Input: part model. Units: mm. Frame: model coordinates. A direction names the side the tool comes from. Coordinates: 2 decimals unless noted, no trailing zeros. Loops run counter-clockwise (first coordinate to the right, second up) from the corner with the lowest first, then second, coordinate; pieces in that order, holes last.
(1) Set-up query: faces 1 (the face through (-69.1, 19.27, -19.52)), 2 (the face through (62.2, 10, -26.2)). Return all of +Z, -Z, +X, -X, +Y, -Y with unobstructed straight access to the full face (end or side cutting, diameter ignored); none if empty.
(2) Line query: L1, parallel to X at y = 2.75, z = 24; L2, parallel to X at y = 2.5, z = 26; L3, parallel to Z at x = -60, y = 17.5. Output: solid intervals per line, ascending.
(3) Section B-B, the plane x = 43. Return loops of the section in (y, z).
(4) Mould query, pull axis Z, two halves, no side actions, for faces 3 (the face through (69.1, 29.14, 0.12)), 4 (the face through (60, 14, 19)), 5 (the face through (-57.8, 10, -26.2)), 6 (the face through (-1, 20, -20)). Classes: released by +Z, released by -Z, zero draft, split by the parting line, or undercut.
(5) Contact query for flat-ended pins moving along their axis: P1, Ø6, axis at x = 60, z = -24, coming from the +Y side; P2, Ø3, axis at x = -25, z = 17, coming from the +Y side; P3, Ø5, axis at x = 41.5, y = 14, coming from the -Z side; P4, Ø6, axis at x = -38, z = -5, coming from the -Y side. Output: stop coordinate, or through.
(6) Section A-A, the plane x = 60. Return loops of the section in (y, z).
(7) Section C-C, the plane z = 24. Give the number of separate pieces and of enclosed holes in the cut face, then the cut area to 3 significant figures.
```python
from build123d import *

# Parameters (mm, degrees)
SKETCH1_R           = 2.75
SKETCH1_W           = 130
SKETCH1_H           = 38
BOSS_EXTRUDE1_DEPTH = 10
SKETCH2_W           = 20
SKETCH2_H           = 20
BOSS_EXTRUDE3_DEPTH = 140
SKETCH3_R           = 5
CUT_EXTRUDE1_DEPTH  = 79.74007874
FILLET1_R           = 3


with BuildPart() as part:
    # Sketch1 → Boss-Extrude1 (new body)
    # profile 1 of 6: a face of its own
    with BuildSketch(Plane(origin=(0, 0, 0), x_dir=(1, 0, 0), z_dir=(0, 1, 0))):
        with BuildLine():
            Line((70, 30), (67, 30))
            ThreePointArc((67, 30), (69.121320344, 29.121320344), (70, 27))
            Line((70, 27), (70, 30))
        make_face()
    # profile 2 of 6: a face of its own
    with BuildSketch(Plane(origin=(0, 0, 0), x_dir=(1, 0, 0), z_dir=(0, 1, 0))):
        with BuildLine():
            ThreePointArc((70, 27), (69.121320344, 29.121320344), (67, 30))
            Line((67, 30), (-67, 30))
            ThreePointArc((-67, 30), (-69.121320344, 29.121320344), (-70, 27))
            Line((-70, 27), (-70, -27))
            ThreePointArc((-70, -27), (-69.121320344, -29.121320344), (-67, -30))
            Line((-67, -30), (67, -30))
            ThreePointArc((67, -30), (69.121320344, -29.121320344), (70, -27))
            Line((70, -27), (70, 27))
        make_face()
        with Locations(Location((-60, -24, 0), (0, 0, 270))):
            Circle(SKETCH1_R, mode=Mode.SUBTRACT)
        with Locations(Location((60, 24, 0), (0, 0, 270))):
            Circle(SKETCH1_R, mode=Mode.SUBTRACT)
        with Locations(Location((60, -24, 0), (0, 0, 270))):
            Circle(SKETCH1_R, mode=Mode.SUBTRACT)
        with Locations(Location((-60, 24, 0), (0, 0, 270))):
            Circle(SKETCH1_R, mode=Mode.SUBTRACT)
        Rectangle(SKETCH1_W, SKETCH1_H, mode=Mode.SUBTRACT)
    # profile 3 of 6: a face of its own
    with BuildSketch(Plane(origin=(0, 0, 0), x_dir=(1, 0, 0), z_dir=(0, 1, 0))):
        with BuildLine():
            Line((70, -30), (70, -27))
            ThreePointArc((70, -27), (69.121320344, -29.121320344), (67, -30))
            Line((67, -30), (70, -30))
        make_face()
    # profile 4 of 6: a face of its own
    with BuildSketch(Plane(origin=(0, 0, 0), x_dir=(1, 0, 0), z_dir=(0, 1, 0))):
        with BuildLine():
            ThreePointArc((-70, 27), (-69.121320344, 29.121320344), (-67, 30))
            Line((-67, 30), (-70, 30))
            Line((-70, 30), (-70, 27))
        make_face()
    # profile 5 of 6: a face of its own
    with BuildSketch(Plane(origin=(0, 0, 0), x_dir=(1, 0, 0), z_dir=(0, 1, 0))):
        with BuildLine():
            ThreePointArc((-67, -30), (-69.121320344, -29.121320344), (-70, -27))
            Line((-70, -27), (-70, -30))
            Line((-70, -30), (-67, -30))
        make_face()
    # profile 6 of 6: a face of its own
    with BuildSketch(Plane(origin=(0, 0, 0), x_dir=(1, 0, 0), z_dir=(0, 1, 0))):
        Rectangle(SKETCH1_W, SKETCH1_H)
    extrude(amount=BOSS_EXTRUDE1_DEPTH)

    # Sketch2 → Boss-Extrude3 (add, through all)
    with BuildSketch(Plane.ZY.offset(70)):
        Polygon((-10, 10), (-10, 30), (-30, 10), align=None)
        with Locations((0, 20)):
            Rectangle(SKETCH2_W, SKETCH2_H)
        Polygon((30, 10), (10, 30), (10, 10), align=None)
    extrude(amount=-BOSS_EXTRUDE3_DEPTH)

    # Sketch3 → Cut-Extrude1 (cut, through all)
    with BuildSketch(Plane(origin=(0, 10, 0), x_dir=(1, 0, 0), z_dir=(0, 1, 0))):
        with Locations(Location((60, 24, 0), (0, 0, 90))):
            Circle(SKETCH3_R)
        with Locations(Location((60, -24, 0), (0, 0, 270))):
            Circle(SKETCH3_R)
        with Locations(Location((-60, 24, 0), (0, 0, 90))):
            Circle(SKETCH3_R)
        with Locations(Location((-60, -24, 0), (0, 0, 270))):
            Circle(SKETCH3_R)
    extrude(amount=CUT_EXTRUDE1_DEPTH, mode=Mode.SUBTRACT)

    # Fillet1
    fillet1_edges = [part.edges().sort_by_distance(p)[0] for p in [
        (0, 10, -30),
        (70, 5, 30),
        (-70, 5, 30),
        (-70, 5, -30),
        (70, 5, -30),
        (0, 10, 30),
        (-70, 20, -20),
        (70, 30, 0),
        (0, 30, -10),
        (-70, 20, 20),
        (0, 30, 10),
        (70, 20, -20),
        (70, 20, 20),
        (-70, 30, 0),
    ]]
    fillet(fillet1_edges, radius=FILLET1_R)


solid = part.part
```
Report:
1. face 1: -Z, -X, +Y
1. face 2: +Y
2. L1: x = -70 to -62.75, -57.25 to 57.25, 62.75 to 70
2. L2: x = -70 to -61.89, -58.11 to 58.11, 61.89 to 70
2. L3: z = -19 to 19
3. outline: (0, -30) - (8.76, -30) arc R3 ccw to (10.88, -29.12) - (29.12, -10.88) arc R3 ccw to (30, -8.76) - (30, 8.76) arc R3 ccw to (29.12, 10.88) - (10.88, 29.12) arc R3 ccw to (8.76, 30) - (0, 30) - close
4. face 3: zero draft
4. face 4: undercut
4. face 5: undercut
4. face 6: released by -Z
5. P1: stops at y = 10
5. P2: stops at y = 24.5
5. P3: stops at z = -28.5
5. P4: stops at y = 0
6. outline: (0, -30) - (8.76, -30) arc R3 ccw to (10.88, -29.12) - (11, -29) - (10, -29) - (10, -26.75) - (0, -26.75) - close; (0, -21.25) - (10, -21.25) - (10, -19) - (21, -19) - (29.12, -10.88) arc R3 ccw to (30, -8.76) - (30, 8.76) arc R3 ccw to (29.12, 10.88) - (21, 19) - (10, 19) - (10, 21.25) - (0, 21.25) - close; (0, 26.75) - (10, 26.75) - (10, 29) - (11, 29) - (10.88, 29.12) arc R3 ccw to (8.76, 30) - (0, 30) - close
7. separate pieces: 3
7. enclosed holes: 0
7. area: 2,000 mm2
